Here's how the part is built. I have some questions about the finished solid (model axes, mm). A direction names the side the tool comes from. Round coordinates to 2 decimals unless told otherwise and drop trailing zeros. Order: outer loops, then holes, each group sorted by start corner. A loop starts at its lowest first (then second) coordinate and runs counter-clockwise, first axis right, second up. Notation, with made-up numbers: (79.25, -34.75) -> (103.25, -34.75) arc R27 cw to (103.25, -18.75) -> close; hole circle Ø2 at (31, 33.5). An arc over 180 degrees is marked (long way). Use a Markdown table: item, result. Add a question column.
(1) I'm going to push flat-ended pins straight in: P1, Ø6, axis at x = 96, y = 284.5, coming from the -Z side; P2, Ø1, axis at x = -154.5, y = -122, coming from the +Z side. Where does each tip first touch, or does it pass through?
(2) I want a section at C-C, the plane z = 830.5. Please give me the cut outline in (x, y), then the cut area to 3 significant figures.
(3) I want a section at A-A, the plane z = 172. Please give me the cut outline in (x, y).
(4) I want a section at B-B, the plane y = -209. Please give me the cut outline in (x, z).
(5) On a 3-axis mill with a long thin cutter (end or side, diameter ignored), from which of +Z, -Z, +X, -X, +Y, -Y can I reach the whole of each face in a straight line? I mean faces 1 (the face through (-2, 349.286, 714)), 2 (the face through (-105, -412.714, 451)), 3 (the face through (-380, 349.286, 213)), 4 (the face through (307.367, 424, 213)). Say none if no direction works.
(6) I want a section at D-D, the plane x = 210. Please give me the cut outline in (y, z), then the cut area to 3 significant figures.
(7) Thinking about a two-plate mould opening in X: for faces 5 (the face through (459.767, 38, 552)), 6 (the face through (-4, 501.686, 552)), 7 (the face through (-454.633, 38, 552)), 8 (the face through (-302.233, 424, 213)), which applies, pulls with the +X half, pulls with the -X half, needs draft (parallel to the pull), parting line crosses it, or undercut?
(8) If I drill on probe 1 along X at (y, z) = (-131, 740); probe 2 along Y at (x, z) = (397, 391.5); probe 3 along Y at (x, z) = (201, 792), over which ranges is the centre line in solid material (lowest first)?
from build123d import *

# Parameters (mm, degrees)
F0_W     = 914.4
F0_H     = 914.4
F1_DEPTH = 914.4
F2_W     = 609.6
F2_H     = 762
F3_DEPTH = 406.4
F4_W     = 609.6
F4_H     = 431.8
F5_DEPTH = 914.401
F6_W     = 609.6
F6_H     = 431.8
F7_DEPTH = 914.401


with BuildPart() as f1:
    # F0 (on Top) → F1 (new body)
    with BuildSketch(Plane.XY):
        with Locations((2.566727, 44.486442)):
            Rectangle(F0_W, F0_H)
    extrude(amount=F1_DEPTH)

    # F2 (on face) → F3 (cut)
    with BuildSketch(Plane.XY.offset(914.4)):
        with Locations((2.566727, -31.713558)):
            Rectangle(F2_W, F2_H)
    extrude(amount=-F3_DEPTH, mode=Mode.SUBTRACT)

    # F4 (on face) → F5 (cut, through all)
    with BuildSketch(Plane.XZ.offset(412.713558)):
        with Locations((2.566727, 215.9)):
            Rectangle(F4_W, F4_H)
    extrude(amount=-F5_DEPTH, mode=Mode.SUBTRACT)

    # F6 (on face) → F7 (cut, through all)
    with BuildSketch(Plane(origin=(-454.633273, 0, 0), x_dir=(0, -1, 0), z_dir=(-1, 0, 0))):
        with Locations((-44.486442, 215.9)):
            Rectangle(F6_W, F6_H)
    extrude(amount=-F7_DEPTH, mode=Mode.SUBTRACT)


solid = f1.part
Taken from the geometry:
| question | item | result |
|---|---|---|
| 1 | P1 | stops at z = 431.8 |
| 1 | P2 | stops at z = 508 |
| 2 | outline | (-454.63, -412.71) -> (-302.23, -412.71) -> (-302.23, 349.29) -> (307.37, 349.29) -> (307.37, -412.71) -> (459.77, -412.71) -> (459.77, 501.69) -> (-454.63, 501.69) -> close |
| 2 | area | 372,000 mm2 |
| 3 | outline | (-454.63, -412.71) -> (-302.23, -412.71) -> (-302.23, -260.31) -> (-454.63, -260.31) -> close; (-454.63, 349.29) -> (-302.23, 349.29) -> (-302.23, 501.69) -> (-454.63, 501.69) -> close; (307.37, -412.71) -> (459.77, -412.71) -> (459.77, -260.31) -> (307.37, -260.31) -> close; (307.37, 349.29) -> (459.77, 349.29) -> (459.77, 501.69) -> (307.37, 501.69) -> close |
| 4 | outline | (-454.63, 431.8) -> (459.77, 431.8) -> (459.77, 914.4) -> (307.37, 914.4) -> (307.37, 508) -> (-302.23, 508) -> (-302.23, 914.4) -> (-454.63, 914.4) -> close |
| 5 | face 1 | +Z, -Y |
| 5 | face 2 | +Z, -Z, +X, -X, -Y |
| 5 | face 3 | -Z, +X, -X |
| 5 | face 4 | -Z, +Y, -Y |
| 6 | outline | (-412.71, 431.8) -> (501.69, 431.8) -> (501.69, 914.4) -> (349.29, 914.4) -> (349.29, 508) -> (-412.71, 508) -> close |
| 6 | area | 132,000 mm2 |
| 7 | face 5 | pulls with the +X half |
| 7 | face 6 | needs draft |
| 7 | face 7 | pulls with the -X half |
| 7 | face 8 | undercut |
| 8 | probe 1 | x = -454.63 to -302.23, 307.37 to 459.77 |
| 8 | probe 2 | y = -412.71 to -260.31, 349.29 to 501.69 |
| 8 | probe 3 | y = 349.29 to 501.69 |
